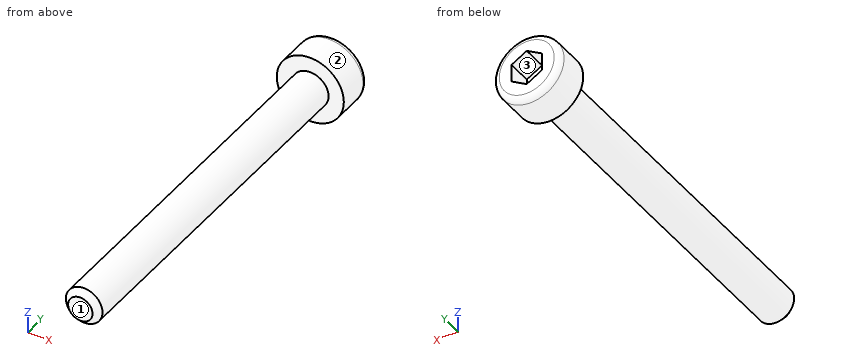
```python
from build123d import *

# Parameters (mm, degrees)
CORTAR_EXTRUIR1_DEPTH = 2
CHAFL_N1_SIZE         = 0.5
REDONDEO1_R           = 0.5


with BuildPart() as part:
    # Croquis1 → Revolución1 (revolve)
    with BuildSketch(Plane.XY):
        Polygon((0, 0), (2.75, 0), (2.75, -3), (1.5, -3), (1.5, -33), (0, -33), align=None)
    revolve(axis=Axis((0, 0, 0), (0, -1, 0)))

    # Croquis2 → Cortar-Extruir1 (cut)
    with BuildSketch(Plane(origin=(0, 0, 0), x_dir=(1, 0, 0), z_dir=(0, 1, 0))):
        Polygon((1.25, 0.721687836), (0, 1.443375673), (-1.25, 0.721687836), (-1.25, -0.721687836), (0, -1.443375673), (1.25, -0.721687836), align=None)
    extrude(amount=-CORTAR_EXTRUIR1_DEPTH, mode=Mode.SUBTRACT)

    # Chaflán1
    chafl_n1_edges = [part.edges().sort_by_distance(p)[0] for p in [
        (-1.5, -33, 0),
    ]]
    chamfer(chafl_n1_edges, length=CHAFL_N1_SIZE)

    # Redondeo1
    redondeo1_edges = [part.edges().sort_by_distance(p)[0] for p in [
        (-2.75, 0, 0),
    ]]
    fillet(redondeo1_edges, radius=REDONDEO1_R)


solid = part.part
```
Geometry: final body of the model. Coordinates: model frame, mm. Face numbers are marked on the shaded views. Round coordinates to 2 decimals unless told otherwise and drop trailing zeros. Loops run counter-clockwise (first coordinate to the right, second up) from the corner with the lowest first, then second, coordinate; pieces in that order, holes last. Notation, with made-up numbers: (-14.75, 23) -> (42.25, 23) arc R21 ccw to (42.25, 54) -> close; hole circle Ø3 at (10, 2). An arc over 180 degrees is marked (long way). Use one line per item in the form item = value.
Item 1: Material intervals for probe 1 along Z at (x, y) = (-1, -1.5); probe 2 along Y at (x, z) = (0.05, 2.3); probe 3 along X at (y, z) = (-28, 0.15), sorted ascending.
Evaluation:
probe_1 = -2.56 to -0.87, 0.87 to 2.56
probe_2 = -3 to 0
probe_3 = -1.49 to 1.49
Item 2: Cut plane A-A on z = 0. Output: boundary loops of the cut face in (x, y).
Evaluation:
outline = (-2.75, -3) -> (-1.5, -3) -> (-1.5, -32.5) -> (-1, -33) -> (1, -33) -> (1.5, -32.5) -> (1.5, -3) -> (2.75, -3) -> (2.75, -0.5) arc R0.5 ccw to (2.25, 0) -> (1.25, 0) -> (1.25, -2) -> (-1.25, -2) -> (-1.25, 0) -> (-2.25, 0) arc R0.5 ccw to (-2.75, -0.5) -> close
Item 3: Cut plane B-B on y = -10. Output: boundary loops of the cut face in (x, z), then the cut area to 3 significant figures.
Evaluation:
outline = circle Ø3 at (0, 0)
area = 7.07 mm2
Item 4: Contact query for flat-ended pins moving along their axis: pin 1 Ø3 at (y, z) = (-11, -0.5) entering from +X; pin 2 Ø3 at (y, z) = (-24.5, -1.5) entering from -X. Output: stop coordinate, or through.
Evaluation:
pin_1 = 1.5
pin_2 = -1.5
Item 5: Draft query along X for the marked faces 1, 2 and 3. Return one class per face: released by +X, released by -X, zero draft, split by the parting line, or undercut.
Evaluation:
face_1 = zero draft
face_2 = split by the parting line
face_3 = undercut
